```python
from build123d import *

# Parameters (mm, degrees)
SKETCH1_W           = 61
SKETCH1_H           = 27
BOSS_EXTRUDE1_DEPTH = 3
SKETCH2_W           = 5
SKETCH2_H           = 27
BOSS_EXTRUDE2_DEPTH = 7
SKETCH3_W           = 15
SKETCH3_H           = 27
BOSS_EXTRUDE3_DEPTH = 5
CUT_EXTRUDE1_DEPTH  = 77.615925238
FILLET1_R           = 2
FILLET2_R           = 2
FILLET3_R           = 1


with BuildPart() as part:
    # Sketch1 → Boss-Extrude1 (new body)
    with BuildSketch(Plane(origin=(0, 0, 0), x_dir=(1, 0, 0), z_dir=(0, 1, 0))):
        with Locations((30.5, 13.5)):
            Rectangle(SKETCH1_W, SKETCH1_H)
    extrude(amount=BOSS_EXTRUDE1_DEPTH)

    # Sketch2 → Boss-Extrude2 (add)
    with BuildSketch(Plane(origin=(0, 3, 0), x_dir=(1, 0, 0), z_dir=(0, 1, 0))):
        with Locations((2.5, 13.5)):
            Rectangle(SKETCH2_W, SKETCH2_H)
        with Locations((58.5, 13.5)):
            Rectangle(SKETCH2_W, SKETCH2_H)
    extrude(amount=BOSS_EXTRUDE2_DEPTH)

    # Sketch3 → Boss-Extrude3 (add)
    with BuildSketch(Plane(origin=(0, 10, 0), x_dir=(1, 0, 0), z_dir=(0, 1, 0))):
        with Locations((-2.5, 13.5)):
            Rectangle(SKETCH3_W, SKETCH3_H)
        with Locations((63.5, 13.5)):
            Rectangle(SKETCH3_W, SKETCH3_H)
    extrude(amount=BOSS_EXTRUDE3_DEPTH)

    # Sketch4 → Cut-Extrude1 (cut, through all)
    with BuildSketch(Plane.XZ.offset(-10)):
        with BuildLine():
            Line((-3.65, -4.35), (-3.65, -22.65))
            ThreePointArc((-3.65, -22.65), (-5, -24), (-6.35, -22.65))
            Line((-6.35, -22.65), (-6.35, -4.35))
            ThreePointArc((-6.35, -4.35), (-5, -3), (-3.65, -4.35))
        make_face()
        with BuildLine():
            Line((67.35, -4.35), (67.35, -22.65))
            ThreePointArc((67.35, -22.65), (66, -24), (64.65, -22.65))
            Line((64.65, -22.65), (64.65, -4.35))
            ThreePointArc((64.65, -4.35), (66, -3), (67.35, -4.35))
        make_face()
    extrude(amount=-CUT_EXTRUDE1_DEPTH, mode=Mode.SUBTRACT)

    # Fillet1
    fillet1_edges = [part.edges().sort_by_distance(p)[0] for p in [
        (-10, 12.5, -27),
        (-10, 12.5, 0),
        (71, 12.5, 0),
        (71, 12.5, -27),
    ]]
    fillet(fillet1_edges, radius=FILLET1_R)

    # Fillet2
    fillet2_edges = [part.edges().sort_by_distance(p)[0] for p in [
        (5, 15, -13.5),
        (56, 15, -13.5),
        (61, 0, -13.5),
        (0, 0, -13.5),
    ]]
    fillet(fillet2_edges, radius=FILLET2_R)

    # Fillet3
    fillet3_edges = [part.edges().sort_by_distance(p)[0] for p in [
        (5, 3, -13.5),
        (56, 3, -13.5),
    ]]
    fillet(fillet3_edges, radius=FILLET3_R)


solid = part.part
```
Geometry: final body of the model. Coordinates: model frame, mm. A direction names the side the tool comes from. Round coordinates to 2 decimals unless told otherwise and drop trailing zeros. Write each loop counter-clockwise with the first axis right and the second up, starting at its lowest first coordinate (ties: lowest second). Pieces come first, ordered by that corner, then holes. Notation, with made-up numbers: (-35.5, 17) -> (-6.5, 17) arc R24 ccw to (-6.5, 56) -> close; hole circle Ø4 at (-3.5, 82). An arc over 180 degrees is marked (long way). Use CSV: the item, a comma, the result in double quotes. Start each with the question number.
Q1. First-contact query: pin 1 Ø8 at (x, z) = (-3.5, -18.5) entering from -Y; pin 2 Ø8 at (x, z) = (38, -11) entering from +Y; pin 3 Ø8 at (x, z) = (67, -12.5) entering from -Y; pin 4 Ø1.5 at (x, y) = (21.5, 5.5) entering from +Z. Flat tips, straight axial feed; report the tip coordinate or a pass-through.
Q2. Section C-C (x = -5). Return loops of the section in (y, z), plus the area to 3 significant figures.
Q3. Line query: L1, parallel to X at y = 11.25, z = -14.25; L2, parallel to X at y = 6.75, z = -25; L3, parallel to X at y = 12.75, z = -3.75. Output: solid intervals per line, ascending.
Q4. Reachability of faces 1 (the face through (5, 8, -13)), 2 (the face through (0, 6, -13)), 3 (the face through (71, 12, -13)), 4 (the face through (64, 15, -14)), 5 (the face through (-5, 12, -3)) from +Z, -Z, +X, -X, +Y, -Y: full face, straight path, thin tool, end or side. Return the list, or none.
Q5. Section A-A (y = 8). Return loops of the section in (x, z).
Q6. Section B-B (z = -10.75). Return loops of the section in (x, y), plus the area to 3 significant figures.
Q7. Section D-D (x = 48.5). Return loops of the section in (y, z), plus the area to 3 significant figures.
Q8. Pull-direction query (X, two-part tool) for faces 6 (the face through (64, 10, -14)), 7 (the face through (60.4, 0.57, -13.69)), 8 (the face through (66, 12, -24)); classes: pulls with the +X half, pulls with the -X half, needs draft (parallel to the pull), parting line crosses it, or undercut.
Result sheet:
1,pin 1,"y = 0.68"
1,pin 2,"y = 3"
1,pin 3,"y = 10"
1,pin 4,"through"
2,outline,"(10, -27) -> (15, -27) -> (15, -24) -> (10, -24) -> close; (10, -3) -> (15, -3) -> (15, 0) -> (10, 0) -> close"
2,area,"30.0 mm²"
3,L1,"-10 to -6.35, -3.65 to 5, 56 to 64.65, 67.35 to 71"
3,L2,"0 to 5, 56 to 61"
3,L3,"-10 to -6.21, -3.79 to 5, 56 to 64.79, 67.21 to 71"
4,face 1,"+Z, -Z, +Y"
4,face 2,"+Z, -Z, -X, -Y"
4,face 3,"+Z, -Z, +X, +Y, -Y"
4,face 4,"+Z, -Z, +X, -X, +Y"
4,face 5,"+Y, -Y"
5,outline,"(0, -27) -> (5, -27) -> (5, 0) -> (0, 0) -> close; (56, -27) -> (61, -27) -> (61, 0) -> (56, 0) -> close"
6,outline,"(-10, 10) -> (-6.35, 10) -> (-6.35, 15) -> (-10, 15) -> close; (-3.65, 10) -> (0, 10) -> (0, 2) arc R2 ccw to (2, 0) -> (59, 0) arc R2 ccw to (61, 2) -> (61, 10) -> (64.65, 10) -> (64.65, 15) -> (58, 15) arc R2 ccw to (56, 13) -> (56, 4) arc R1 cw to (55, 3) -> (6, 3) arc R1 cw to (5, 4) -> (5, 13) arc R2 ccw to (3, 15) -> (-3.65, 15) -> close; (67.35, 10) -> (71, 10) -> (71, 15) -> (67.35, 15) -> close"
6,area,"373 mm²"
7,outline,"(0, -27) -> (3, -27) -> (3, 0) -> (0, 0) -> close"
7,area,"81.0 mm²"
8,face 6,"needs draft"
8,face 7,"pulls with the +X half"
8,face 8,"undercut"
